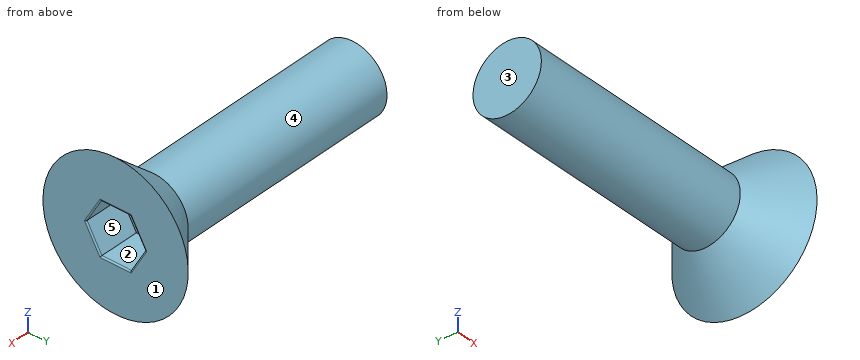
from build123d import *

# Parameters (mm, degrees)
CUT_EXTRUDE1_DEPTH = 3.81
FILLET1_R          = 0.127


with BuildPart() as part:
    # Sketch1 → Revolve1 (revolve)
    with BuildSketch(Plane(origin=(0, 0, 0), x_dir=(1, 0, 0), z_dir=(0, 1, 0)), mode=Mode.PRIVATE) as revolve1_sk:
        Polygon((0, 0), (0, 6.7437), (-4.105319735, 3.175), (-25.4, 3.175), (-25.4, 0), align=None)
    revolve(revolve1_sk.sketch.rotate(Axis((-25.4, 0, 0), (1, 0, 0)), 180), axis=Axis((-25.4, 0, 0), (1, 0, 0)))

    # Sketch2 → Cut-Extrude1 (cut)
    with BuildSketch(Plane(origin=(0, 0, 0), x_dir=(0, 0, -1), z_dir=(1, 0, 0))):
        Polygon((0, 2.749630657), (-2.38125, 1.374815329), (-2.38125, -1.374815329), (0, -2.749630657), (2.38125, -1.374815329), (2.38125, 1.374815329), align=None)
    extrude(amount=-CUT_EXTRUDE1_DEPTH, mode=Mode.SUBTRACT)

    # Fillet1
    fillet1_edges = [part.edges().sort_by_distance(p)[0] for p in [
        (0, 2.062222993, -1.190625),
        (0, 2.062222993, 1.190625),
        (0, 0, 2.38125),
        (0, -2.062222993, 1.190625),
        (0, -2.062222993, -1.190625),
        (0, 0, -2.38125),
    ]]
    fillet(fillet1_edges, radius=FILLET1_R)


solid = part.part
Could you check a few things on this model? Use its own coordinates, in mm. Face numbers are marked on the shaded views. A direction names the side the tool comes from. Coordinates: 2 decimals unless noted, no trailing zeros. Write each loop counter-clockwise with the first axis right and the second up, starting at its lowest first coordinate (ties: lowest second). Pieces come first, ordered by that corner, then holes. Notation, with made-up numbers: (61.5, -18.5) - (99.5, -18.5) arc R11 ccw to (99.5, 2.5) - close; hole circle Ø7 at (-19.75, 37). An arc over 180 degrees is marked (long way). Put each result on its own line as item: value. Start each with the question number.
Q1. I want a section at A-A on y = 0. Write out the boundary of the cut face in (x, z) (3 decimals).
Q2. Which directions (+Z, -Z, +X, -X, +Y, -Y) give clear straight access to the entire face, cutting with the end or side of a thin tool? Please do the marked faces 1 and 2.
Q3. Thinking about a two-plate mould opening in Y: for the marked faces 3, 4 and 5, which applies, pulls with the +Y half, pulls with the -Y half, needs draft (parallel to the pull), parting line crosses it, or undercut?
Q4. Please list where these lines run through material, in increasing order: L1, parallel to X at y = 1.75, z = -1.25; L2, parallel to Y at x = -9.5, z = 0 (3 decimals); L3, parallel to Z at x = -1.75, y = 4.5.
Q5. I'm going to push flat-ended pins straight in: P1, Ø4, axis at x = -12.5, y = 1.5, coming from the -Z side (3 decimals); P2, Ø6, axis at x = -19, z = 4, coming from the +Y side; P3, Ø5, axis at y = -2.5, z = 2, coming from the -X side; P4, Ø4, axis at x = -9.5, y = 3.5, coming from the +Z side. Where does each tip first touch, or does it pass through?
Q6. I want a section at B-B on x = -14.5. Write out the boundary of the cut face in (y, z) (3 decimals).
Checks:
1. outline: (-25.4, -3.175) - (-4.105, -3.175) - (0, -6.744) - (0, -2.508) arc R0.127 ccw to (-0.127, -2.381) - (-3.81, -2.381) - (-3.81, 2.381) - (-0.127, 2.381) arc R0.127 ccw to (0, 2.508) - (0, 6.744) - (-4.105, 3.175) - (-25.4, 3.175) - close
2. face 1: +Z, -Z, +X, +Y, -Y
2. face 2: +X
3. face 3: needs draft
3. face 4: parting line crosses it
3. face 5: undercut
4. L1: -25.4 to -3.81
4. L2: -3.175 to 3.175
4. L3: -2.65 to 2.65
5. P1: z = -3.175
5. P2: y = 3.01
5. P3: x = -25.4
5. P4: z = 2.8
6. outline: circle Ø6.35 at (0, 0)
